Build history of the part. All positions in model axes, mm. Coordinates: 2 decimals unless noted, no trailing zeros. Order: outer loops, then holes, each group sorted by start corner. A loop starts at its lowest first (then second) coordinate and runs counter-clockwise, first axis right, second up. Notation, with made-up numbers: M 19,-21.75 L 36,-21.75 A20 cw 36,1.25 Z; hole C 3,62 d5. An arc over 180 degrees is marked long. Write item = value, one per line. Start each with the question number.
Q1. Band-saw the part on C-C on x = 1. Write the cut outline in (y, z).
Q2. Drill centre line: probe 1 along Z at (x, y) = (1.65, -26.5). Where is it in solid material? Low to high.
Q3. Band-saw the part on B-B on z = -72.5. Write the cut outline in (x, y), plus the area to 3 significant figures.
Q4. Band-saw the part on A-A on y = -47. Write the cut outline in (x, z), plus the area to 3 significant figures.
```python
from build123d import *

# Parameters (mm, degrees)
F0_W     = 235
F0_H     = 190
F1_DEPTH = 3
F2_W     = 6
F2_H     = 50
F3_DEPTH = 25


with BuildPart() as f1:
    # F0 (on Right) → F1 (new body)
    with BuildSketch(Plane.YZ):
        Rectangle(F0_W, F0_H)
    extrude(amount=F1_DEPTH)

    # F2 (on face) → F3 (cut)
    with BuildSketch(Plane.YZ.offset(3)):
        with Locations((-64.5, -50)):
            Rectangle(F2_W, F2_H)
        with Locations((-55.5, -50)):
            Rectangle(F2_W, F2_H)
        with Locations((-46.5, -50)):
            Rectangle(F2_W, F2_H)
        with Locations((-37.5, -50)):
            Rectangle(F2_W, F2_H)
        with Locations((-28.5, -50)):
            Rectangle(F2_W, F2_H)
        with Locations((-19.5, -50)):
            Rectangle(F2_W, F2_H)
    extrude(amount=-F3_DEPTH, mode=Mode.SUBTRACT)


solid = f1.part
```
Recorded:
q1.outline = M -117.5,-95 L 117.5,-95 L 117.5,95 L -117.5,95 Z; hole M -67.5,-75 L -61.5,-75 L -61.5,-25 L -67.5,-25 Z; hole M -58.5,-75 L -52.5,-75 L -52.5,-25 L -58.5,-25 Z; hole M -49.5,-75 L -43.5,-75 L -43.5,-25 L -49.5,-25 Z; hole M -40.5,-75 L -34.5,-75 L -34.5,-25 L -40.5,-25 Z; hole M -31.5,-75 L -25.5,-75 L -25.5,-25 L -31.5,-25 Z; hole M -22.5,-75 L -16.5,-75 L -16.5,-25 L -22.5,-25 Z
q2.probe_1 = -95 to -75, -25 to 95
q3.outline = M 0,-117.5 L 3,-117.5 L 3,-67.5 L 0,-67.5 Z; M 0,-61.5 L 3,-61.5 L 3,-58.5 L 0,-58.5 Z; M 0,-52.5 L 3,-52.5 L 3,-49.5 L 0,-49.5 Z; M 0,-43.5 L 3,-43.5 L 3,-40.5 L 0,-40.5 Z; M 0,-34.5 L 3,-34.5 L 3,-31.5 L 0,-31.5 Z; M 0,-25.5 L 3,-25.5 L 3,-22.5 L 0,-22.5 Z; M 0,-16.5 L 3,-16.5 L 3,117.5 L 0,117.5 Z
q3.area = 597 mm2
q4.outline = M 0,-95 L 3,-95 L 3,-75 L 0,-75 Z; M 0,-25 L 3,-25 L 3,95 L 0,95 Z
q4.area = 420 mm2
